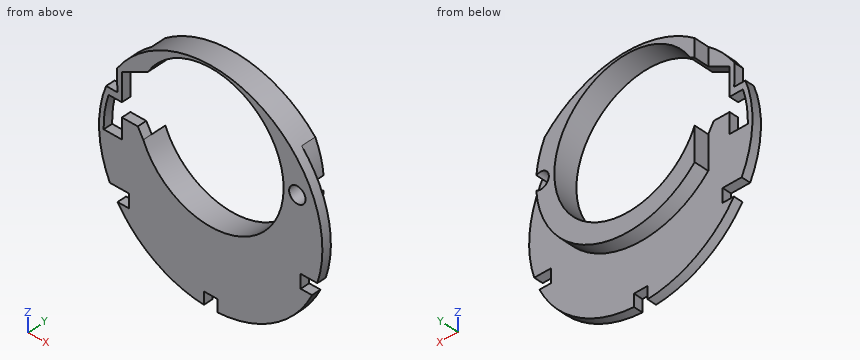
from build123d import *

# Parameters (mm, degrees)
BOSS_EXTRUDE1_DEPTH     = 1
BOSS_EXTRUDE2_DEPTH     = 1.6
CUT_EXTRUDE1_DEPTH      = 18.39784469409933
CUT_EXTRUDE1_DEPTH_BACK = 18.39784469409933
SKETCH2_R               = 0.9000000000000004


with BuildPart() as part:
    # Sketch1 → Boss-Extrude1 (new body)
    with BuildSketch(Plane(origin=(0, 0, 0), x_dir=(1, 0, 0), z_dir=(0, 1, 0))):
        with BuildLine():
            Line((-0.75, 10.875000000000002), (-0.75, 12.227019260637483))
            ThreePointArc((-0.7500000000000002, 12.227019260637485), (-6.131762108207349, 10.604904216840085), (-10.22252415013044, 6.750000000000002))
            Line((-10.222524150130438, 6.750000000000001), (-8.975, 6.750000000000001))
            Line((-8.975, 6.750000000000001), (-8.975, 5.249999999999999))
            Line((-8.975, 5.249999999999999), (-11.067971810589329, 5.249999999999999))
            ThreePointArc((-11.06797181058933, 5.25), (-12.238613585290821, 0.528050669855673), (-11.479034225714315, -4.277180525168357))
            Line((-11.479034225714315, -4.277180525168356), (-10.251454558987772, -4.277180525168356))
            Line((-10.251454558987772, -4.277180525168356), (-10.261976170759779, -6.689868838083338))
            ThreePointArc((-10.26197617075978, -6.68986883808334), (5.219252819608776, -11.082504229866366), (11.693587986584786, 3.65))
            Line((11.693587986584786, 3.6499999999999995), (9.875, 3.6499999999999995))
            Line((9.875, 3.6499999999999995), (9.875, 5.1499999999999995))
            Line((9.875, 5.1499999999999995), (11.114854924829205, 5.1499999999999995))
            ThreePointArc((11.114854924829206, 5.15), (6.9075861196708574, 10.116706677537433), (0.7500000000000135, 12.227019260637483))
            Line((0.7500000000000137, 12.227019260637483), (0.7500000000000137, 10.875000000000002))
            Line((0.7500000000000137, 10.875000000000002), (-0.7500000000000001, 10.875000000000002))
        make_face()
    extrude(amount=BOSS_EXTRUDE1_DEPTH)

    # Sketch3 → Boss-Extrude2 (add)
    with BuildSketch(Plane(origin=(0, 1, 0), x_dir=(1, 0, 0), z_dir=(0, 1, 0))):
        with BuildLine():
            Line((-7.4007200688618315, 2.7252763855729887), (-7.4007200688618315, -0.9620167113123034))
            ThreePointArc((-7.40072006886183, -0.9620167113123008), (1.5482634545040064, 3.8487502365311173), (8, -4.0000000000000036))
            ThreePointArc((8, -4.000000000000005), (1.5482634545039802, -11.84875023653113), (-7.400720068861849, -7.037983288687658))
            Line((-7.400720068861849, -7.037983288687658), (-7.400720068861849, -9.761754066884983))
            ThreePointArc((-7.400720068861847, -9.761754066884983), (1.1153735220053107, -12.199116439579116), (9.048261308939445, -8.257812499999588))
            ThreePointArc((9.048261308939306, -8.257812499999497), (9.759165258601607, -6.181442975487434), (10, -4.000000000000006))
            ThreePointArc((10, -4.0000000000000036), (3.6050519629668107, 5.327572049805301), (-7.400720068861829, 2.7252763855729913))
        make_face()
    extrude(amount=BOSS_EXTRUDE2_DEPTH)

    # Sketch2 → Cut-Extrude1 (cut, two sides: drawn at the far end of the back side and taken through both)
    with BuildSketch(Plane(origin=(0, 1, 0), x_dir=(1, 0, 0), z_dir=(0, 1, 0)).offset(-CUT_EXTRUDE1_DEPTH_BACK)):
        with BuildLine():
            Line((-8.000000000000002, -2.0000000000000036), (-9.747973362219389, -2.0000000000000036))
            Line((-9.747973362219389, -2.0000000000000036), (-9.747973362219389, 0.22281947483164366))
            Line((-9.747973362219389, 0.22281947483164363), (-11.742905111754867, 0.22281947483164344))
            ThreePointArc((-11.742905111754867, 0.22281947483164347), (-11.62509617448331, -1.6740991356715729), (-11.202877600193457, -3.5271805251683066))
            Line((-11.202877600193467, -3.5271805251683563), (-9.747973362219389, -3.5271805251683563))
            Line((-9.747973362219389, -3.5271805251683563), (-9.747973362219389, -6.551525342353796))
            Line((-9.747973362219389, -6.551525342353796), (-6.906384460645114, -8.037555409125643))
            ThreePointArc((-6.906384460645114, -8.037555409125643), (7.980546470676243, -3.4424356275935972), (-7.400720068861833, -0.9620167113123106))
            Line((-7.400720068861836, -0.9620167113123133), (-8.000000000000002, -2.0000000000000036))
        make_face()
        with Locations(Location((9.5, -4.1, 0), (0, 0, 270))):
            Circle(SKETCH2_R)
    extrude(amount=CUT_EXTRUDE1_DEPTH + CUT_EXTRUDE1_DEPTH_BACK, mode=Mode.SUBTRACT)


solid = part.part
Work out the finished part from the listing and answer in its coordinate system (mm). Coordinates: 2 decimals unless noted, no trailing zeros. Write each loop counter-clockwise with the first axis right and the second up, starting at its lowest first coordinate (ties: lowest second). Pieces come first, ordered by that corner, then holes. Notation, with made-up numbers: M 45,-30 L 59,-30 A23 ccw 59,-6 Z; hole C 39,-21 d3. An arc over 180 degrees is marked long. Use one line per item in the form item = value. Start each with the question number.
1. Straight lines are drawn through the part: probe 1 along Z at (x, y) = (0, 0.7) (3 decimals); probe 2 along X at (y, z) = (0.4, 4.5); probe 3 along X at (y, z) = (0.9, 4). For each, find the intervals that lie inside material, in ascending order. Write a range as from..to.
2. The part is cut by section B-B (y = 0.55). Give the vertices of the cut face in (x, z) (3 decimals), plus the area to 3 significant figures.
3. The part is cut by section C-C (y = 2.3). Give the vertices of the cut face in (x, z).
4. The part is cut by section D-D (x = 4). Give the vertices of the cut face in (y, z).
5. Each of these flat-tipped pins is pushed along its axis until it touches: P1, Ø0.8, axis at x = -10, y = 0.5, coming from the -Z side; P2, Ø1.1, axis at y = 0.5, z = 5.5, coming from the +X side; P3, Ø0.5, axis at x = -9.5, y = 0.5, coming from the +Z side. Where does it stop, or does it pass through?
6. The part is cut by section A-A (x = 10.75). Give the vertices of the cut face in (y, z).
Evaluation:
q1.probe_1 = -10.875..-4, 12..12.25
q1.probe_2 = -10.25..-9.75, 7.98..8.69, 10.31..11.39
q1.probe_3 = -11.58..-9.75, 8..8.61, 10.39..11.58
q2.outline = M -11.479,4.277 A12.25 ccw -11.068,-5.25 L -8.975,-5.25 L -8.975,-6.75 L -10.223,-6.75 A12.25 ccw -0.75,-12.227 L -0.75,-10.875 L 0.75,-10.875 L 0.75,-12.227 A12.25 ccw 11.115,-5.15 L 9.875,-5.15 L 9.875,-3.65 L 11.694,-3.65 A12.25 ccw -10.262,6.69 L -10.251,4.277 Z; hole M -11.743,-0.223 L -9.748,-0.223 L -9.748,2 L -8,2 L -7.401,0.962 A8 ccw long -6.906,8.038 L -9.748,6.552 L -9.748,3.527 L -11.203,3.527 A11.745 ccw Z; hole C 9.5,4.1 d1.8
q2.area = 242 mm^2
q3.outline = M -7.4,-2.73 A10 ccw 9.98,3.34 A0.9 cw long 9.96,4.87 A10 ccw 9.05,8.26 A12.25 ccw -7.4,9.76 L -7.4,7.78 L -6.91,8.04 A8 cw long -7.4,0.96 Z
q4.outline = M 0,-11.58 L 1,-11.58 L 1,-5.17 L 2.6,-5.17 L 2.6,-2.93 L 0,-2.93 Z; M 0,10.93 L 2.6,10.93 L 2.6,11.58 L 0,11.58 Z
q5.P1 = -7.61
q5.P2 = 11.21
q5.P3 = 8.03
q6.outline = M 0,-5.87 L 1,-5.87 L 1,-5.15 L 0,-5.15 Z; M 0,-3.65 L 1,-3.65 L 1,5.87 L 0,5.87 Z
